Autodesk Inventor part; units mm, degrees
ref_plane "YZ Plane" through (0, 0, 0) normal (1, 0, 0) x (0, 1, 0)
ref_plane "XZ Plane" through (0, 0, 0) normal (0, 1, 0) x (-1, 0, 0)
ref_plane "XY Plane" through (0, 0, 0) normal (0, 0, 1) x (1, 0, 0)
sketch "Sketch1" plane through (0, 0, 0) normal (0, 0, 1) x (1, 0, 0)
  circle A0 centre (0, 0) radius 3
  dimension "d0" = 6
extrude "Extrusion1" add sketch "Sketch1" along normal blind 12.27
sketch "Sketch2" plane through (0, 0, 12.27) normal (0, 0, 1) x (1, 0, 0)
  line L0 (1.46, 2.6208) -> (1.46, -2.6208)
  circle A0 centre (0, 0) radius 3
  point P0 (-3, 0)
  dimension "d3" = 4.46
extrude "Extrusion2" cut sketch "Sketch2" against normal blind 5.3 contours A0 L0 picked at (2.441, 0.367)
chamfer "Chamfer1" distance 0.5 angle 45 2 edges at (-3, 0, 12.27) (1.46, 0, 12.27)
properties part number "PEC12R-4017F-N0024 Shaft"
Design review of the part built by this model. Coordinates are the model's own, in mm. A direction names the side the tool comes from. Round coordinates to 2 decimals unless told otherwise and drop trailing zeros. Order: outer loops, then holes, each group sorted by start corner. A loop starts at its lowest first (then second) coordinate and runs counter-clockwise, first axis right, second up. Notation, with made-up numbers: (-28, 73.25) - (-8, 73.25) arc R24 ccw to (-8, 92.25) - close; hole circle Ø8 at (-36, -4.75). An arc over 180 degrees is marked (long way). Return JSON: item names as keys, results as strings.
Q1. Wall thickness on L1, parallel to Z at x = 1.9, y = 0.8; L2, parallel to X at y = -0.1, z = 4; L3, parallel to X at y = -0.15, z = 9.25: over which ranges is each line inside the solid? List them lowest first. Write a range as [from, to].
Computed values:
{"L1": "z = [0, 6.97]", "L2": "x = [-3, 3]", "L3": "x = [-3, 1.46]"}
Q2. The part is to be moulded in two halves that separate along X. For faces 1 (the cylindrical face through (-2.4, 1.8, 5.8)), 2 (the flat face through (0, 0, 0)), 3 (the flat face through (1.46, 0, 9)), say which applies: pulls with the +X half, pulls with the -X half, needs draft (parallel to the pull), parting line crosses it, or undercut.
Computed values:
{"face 1": "parting line crosses it", "face 2": "needs draft", "face 3": "pulls with the +X half"}
Q3. Consider section A-A on y = 0. Write out the cut boundary in (x, z), plus the area to 3 significant figures.
Computed values:
{"outline": "(-3, 0) - (3, 0) - (3, 6.97) - (1.46, 6.97) - (1.46, 11.77) - (0.96, 12.27) - (-2.5, 12.27) - (-3, 11.77) - close", "area": "65.2 mm2"}
Q4. For pin 1 Ø1 at (x, z) = (-1, 3) entering from +Y; pin 2 Ø0.5 at (x, y) = (2.5, -1) entering from +Z, all flat-tipped, find the tip position at first contact; note any pin that passes through.
Computed values:
{"pin 1": "stops at y = 2.96", "pin 2": "stops at z = 6.97"}
Q5. Consider section B-B on z = 9.5. Write out the cut boundary in (x, y).
Computed values:
{"outline": "(1.46, -2.62) - (1.46, 2.62) arc R3 ccw (long way) to start"}
Q6. Machinability: for faces 4 (the conical face through (-2.64, -0.08, 12.13)), 5 (the flat face through (2, 0, 6.97)), which of the approach directions +Z, -Z, +X, -X, +Y, -Y give a long, thin tool a straight path to every point of the face, cutting with its end or side? Answer none if there is none.
Computed values:
{"face 4": "+Z", "face 5": "+Z, +X, +Y, -Y"}
